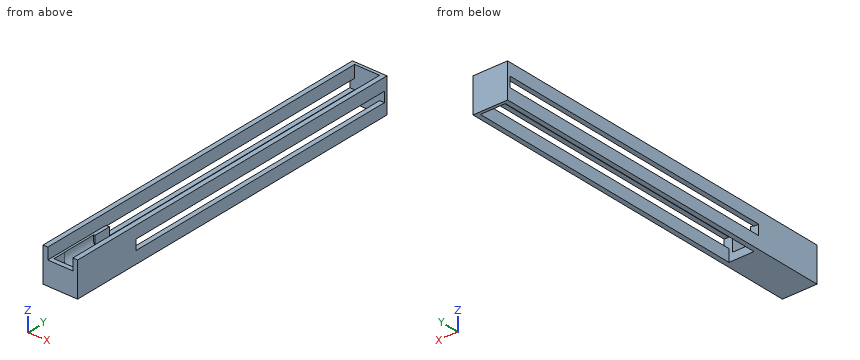
```python
from build123d import *

# Parameters (mm, degrees)
SKETCH1_W           = 22.794602658
SKETCH1_H           = 22.794602658
BOSS_EXTRUDE1_DEPTH = 22.5
SKETCH2_R           = 7.25
CUT_EXTRUDE1_DEPTH  = 11.5
SKETCH4_W           = 16.511455896
SKETCH4_H           = 45
CUT_EXTRUDE2_DEPTH  = 7.5
SKETCH6_W           = 3.141573381
SKETCH6_H           = 8.057746469
BOSS_EXTRUDE2_DEPTH = 192
SKETCH8_W           = 22.794602658
SKETCH8_H           = 22.794602658
BOSS_EXTRUDE3_DEPTH = 2
SKETCH10_W          = 12
SKETCH10_H          = 12.75
CUT_EXTRUDE4_DEPTH  = 11
SKETCH11_W          = 13.5
SKETCH11_H          = 13.5
CUT_EXTRUDE5_DEPTH  = 8


with BuildPart() as part:
    # Sketch1 → Boss-Extrude1 (new, symmetric)
    with BuildSketch(Plane(origin=(0, 0, 0), x_dir=(1, 0, 0), z_dir=(0, 1, 0))):
        Rectangle(SKETCH1_W, SKETCH1_H)
    extrude(amount=BOSS_EXTRUDE1_DEPTH, both=True)

    # Sketch2 → Cut-Extrude1 (cut, symmetric)
    with BuildSketch(Plane(origin=(0, 0, 0), x_dir=(1, 0, 0), z_dir=(0, 1, 0))):
        with Locations(Location((0, -1.5, 0), (0, 0, 270))):
            Circle(SKETCH2_R)
    extrude(amount=CUT_EXTRUDE1_DEPTH, both=True, mode=Mode.SUBTRACT)

    # Sketch4 → Cut-Extrude2 (cut, symmetric)
    with BuildSketch(Plane.XY.offset(11.397301329)):
        Rectangle(SKETCH4_W, SKETCH4_H)
    extrude(amount=CUT_EXTRUDE2_DEPTH, both=True, mode=Mode.SUBTRACT)

    # Sketch6 → Boss-Extrude2 (add)
    with BuildSketch(Plane(origin=(0, 22.5, 0), x_dir=(1, 0, 0), z_dir=(0, 1, 0))):
        with Locations((-9.826514639, 7.368428095)):
            Rectangle(SKETCH6_W, SKETCH6_H)
        with Locations((9.826514639, 7.368428095)):
            Rectangle(SKETCH6_W, SKETCH6_H)
        with Locations((-9.826514639, -7.368428095)):
            Rectangle(SKETCH6_W, SKETCH6_H)
        with Locations((9.826514639, -7.368428095)):
            Rectangle(SKETCH6_W, SKETCH6_H)
    extrude(amount=BOSS_EXTRUDE2_DEPTH)

    # Sketch8 → Boss-Extrude3 (add)
    with BuildSketch(Plane(origin=(0, 214.5, 0), x_dir=(1, 0, 0), z_dir=(0, 1, 0))):
        Rectangle(SKETCH8_W, SKETCH8_H)
    extrude(amount=BOSS_EXTRUDE3_DEPTH)

    # Sketch10 → Cut-Extrude4 (cut)
    with BuildSketch(Plane.XZ.offset(-11.5)):
        Rectangle(SKETCH10_W, SKETCH10_H)
    extrude(amount=-CUT_EXTRUDE4_DEPTH, mode=Mode.SUBTRACT)

    # Sketch11 → Cut-Extrude5 (cut)
    with BuildSketch(Plane(origin=(0, -11.5, 0), x_dir=(1, 0, 0), z_dir=(0, 1, 0))):
        with Locations((0, -1.5)):
            Rectangle(SKETCH11_W, SKETCH11_H)
    extrude(amount=-CUT_EXTRUDE5_DEPTH, mode=Mode.SUBTRACT)


solid = part.part
```
Could you check a few things on this model? Use its own coordinates, in mm. Coordinates: 2 decimals unless noted, no trailing zeros. Write each loop counter-clockwise with the first axis right and the second up, starting at its lowest first coordinate (ties: lowest second). Pieces come first, ordered by that corner, then holes. Notation, with made-up numbers: (-32, 61) -> (25, 61) arc R12 cw to (25, 80) -> close; hole circle Ø11 at (-13.5, 31). An arc over 180 degrees is marked (long way). One line per question, with ' | ' between items. Start each with the question number.
1. If we section it at A-A (x = 0): Please give me the cut outline in (y, z) (3 decimals), and give its area (3 significant figures).
2. Please list where these lines run through material, in increasing order: line 1 along X through (y, z) = (3, 1.5); line 2 along Y through (x, z) = (5.5, 0.75); line 3 along X through (y, z) = (-12, 9.5).
3. Will these pins go through, and if not, where does the flat tip stop? P1, Ø5, axis at x = 3, y = -5, coming from the +Z side; P2, Ø9, axis at x = 2.5, y = -16.5, coming from the +Z side.
4. If we section it at B-B (y = 154.5): Please give me the cut outline in (x, z).
Return value:
1) outline: (-22.5, -11.397) -> (22.5, -11.397) -> (22.5, -6.375) -> (11.5, -6.375) -> (11.5, -5.75) -> (-11.5, -5.75) -> (-11.5, -5.25) -> (-19.5, -5.25) -> (-19.5, 3.897) -> (-22.5, 3.897) -> close; (214.5, -11.397) -> (216.5, -11.397) -> (216.5, 11.397) -> (214.5, 11.397) -> close | area: 326 mm²
2) line 1: x = -11.4 to -7.25, 7.25 to 11.4 | line 2: y = -22.5 to -19.5, 214.5 to 216.5 | line 3: x = -11.4 to -8.26, 8.26 to 11.4
3) P1: stops at z = -3.22 | P2: stops at z = 3.9
4) outline: (-11.4, -11.4) -> (-8.26, -11.4) -> (-8.26, -3.34) -> (-11.4, -3.34) -> close; (-11.4, 3.34) -> (-8.26, 3.34) -> (-8.26, 11.4) -> (-11.4, 11.4) -> close; (8.26, -11.4) -> (11.4, -11.4) -> (11.4, -3.34) -> (8.26, -3.34) -> close; (8.26, 3.34) -> (11.4, 3.34) -> (11.4, 11.4) -> (8.26, 11.4) -> close
